Check sheet for the modelled part. Datum: model origin and axes. Units: mm. A direction names the side the tool comes from. Round coordinates to 2 decimals unless told otherwise and drop trailing zeros. Write each loop counter-clockwise with the first axis right and the second up, starting at its lowest first coordinate (ties: lowest second). Pieces come first, ordered by that corner, then holes.
from build123d import *

# Parameters (mm, degrees)
SKETCH1_W                              = 60
SKETCH1_H                              = 40
BOSS_EXTRUDE1_DEPTH                    = 6.35
SKETCH2_W                              = 6.35
SKETCH2_H                              = 40
BOSS_EXTRUDE2_DEPTH                    = 53.65
FILLET4_R                              = 10
FILLET5_R                              = 10
TAP_DRILL_FOR_M8_HELICOIL1_D           = 8.25
TAP_DRILL_FOR_M8_HELICOIL1_CSINK_D     = 8.3
TAP_DRILL_FOR_M8_HELICOIL1_CSINK_ANGLE = 90
TAP_DRILL_FOR_M8_HELICOIL2_D           = 8.25
TAP_DRILL_FOR_M8_HELICOIL2_CSINK_D     = 8.3
TAP_DRILL_FOR_M8_HELICOIL2_CSINK_ANGLE = 90


with BuildPart() as part:
    # Sketch1 → Boss-Extrude1 (new body)
    with BuildSketch(Plane(origin=(0, 0, 0), x_dir=(1, 0, 0), z_dir=(0, 1, 0))):
        with Locations((11.612905022, -3.595670031)):
            Rectangle(SKETCH1_W, SKETCH1_H)
    extrude(amount=BOSS_EXTRUDE1_DEPTH)

    # Sketch2 → Boss-Extrude2 (add)
    with BuildSketch(Plane(origin=(0, 6.35, 0), x_dir=(1, 0, 0), z_dir=(0, 1, 0))):
        with Locations((38.437905022, -3.595670031)):
            Rectangle(SKETCH2_W, SKETCH2_H)
    extrude(amount=BOSS_EXTRUDE2_DEPTH)

    # Fillet4
    fillet4_edges = [part.edges().sort_by_distance(p)[0] for p in [
        (35.262905022, 6.35, 3.595670031),
    ]]
    fillet(fillet4_edges, radius=FILLET4_R)

    # Fillet5
    fillet5_edges = [part.edges().sort_by_distance(p)[0] for p in [
        (41.612905022, 0, 3.595670031),
    ]]
    fillet(fillet5_edges, radius=FILLET5_R)

    # Tap Drill for M8 Helicoil1 (through all)
    with Locations(Plane(origin=(0, 6.35, 0), x_dir=(1, 0, 0), z_dir=(0, 1, 0))):
        with Locations((12.052905022, -3.595670031), (-5.167094978, -3.595670031)):
            CounterSinkHole(TAP_DRILL_FOR_M8_HELICOIL1_D / 2, TAP_DRILL_FOR_M8_HELICOIL1_CSINK_D / 2, counter_sink_angle=TAP_DRILL_FOR_M8_HELICOIL1_CSINK_ANGLE)

    # Tap Drill for M8 Helicoil2 (through all)
    with Locations(Plane.ZY.offset(-35.262905022)):
        with Locations((3.595670031, 46.78), (3.595670031, 29.56)):
            CounterSinkHole(TAP_DRILL_FOR_M8_HELICOIL2_D / 2, TAP_DRILL_FOR_M8_HELICOIL2_CSINK_D / 2, counter_sink_angle=TAP_DRILL_FOR_M8_HELICOIL2_CSINK_ANGLE)


solid = part.part
1. Sectioned sample at B-B, the plane z = 20. Enter the section's corners in (x, y), plus the area to 3 significant figures.
2. Sectioned sample at D-D, the plane x = 27. Enter the section's corners in (y, z), plus the area to 3 significant figures.
3. Go/stop test with flat-tipped pins: pin 1 (10.5 mm diameter, centred on x = -5.17, z = 3.6, fed in from +Y); pin 2 (3 mm diameter, centred on y = 11, z = 1, fed in from -X). Record where each tip stops, or that it passes through.
4. Set-up check for faces 4 (the flat face through (3, 6.35, 3)), 5 (the flat face through (23, 5, -16.404)): record each of +Z, -Z, +X, -X, +Y, -Y from which the full face is reachable in a straight line by a thin tool's end or side.
5. Sectioned sample at C-C, the plane x = 1.5. Enter the section's corners in (y, z), plus the area to 3 significant figures.
6. Release check for a two-part mould opening along Y. For faces 1 (the flat face through (6, 0, 3)), 2 (the flat face through (23, 5, 23.596)), 3 (the cylindrical face through (38.495, 42.753, 4.49)) record: released by +Y, released by -Y, zero draft, split by the parting line, or undercut.
7. Scan lines: line 1 along X through (y, z) = (27, 9.5); line 2 along Y through (x, z) = (21, -2). Record each from-to range of solid material in increasing order.
Computed values:
1. outline: (-18.39, 0) - (31.61, 0) arc R10 ccw to (41.61, 10) - (41.61, 60) - (35.26, 60) - (35.26, 16.35) arc R10 cw to (25.26, 6.35) - (-18.39, 6.35) - close
1. area: 722 mm2
2. outline: (0, -16.4) - (6.5, -16.4) - (6.5, 23.6) - (0, 23.6) - close
2. area: 260 mm2
3. pin 1: stops at y = 6.35
3. pin 2: stops at x = 32.55
4. face 4: +Z, -Z, -X, +Y
4. face 5: -Z, +X, -X, +Y, -Y
5. outline: (0, -16.4) - (6.35, -16.4) - (6.35, 23.6) - (0, 23.6) - close
5. area: 254 mm2
6. face 1: released by -Y
6. face 2: zero draft
6. face 3: undercut
7. line 1: x = 35.26 to 41.61
7. line 2: y = 0 to 6.35
